from build123d import *
from build123d.topology import SkipClean

# Parameters (mm, degrees)
BOSS_EXTRUDE1_DEPTH     = 10
CUT_EXTRUDE1_DEPTH      = 29.188093475
CUT_EXTRUDE1_DEPTH_BACK = 29.188093475
SKETCH4_R               = 2.05
CUT_EXTRUDE2_OUTLINE_W  = 1.4
CUT_EXTRUDE2_OUTLINE_H  = 5.870544518
CUT_EXTRUDE3_START      = 20
CUT_EXTRUDE3_DEPTH      = 12
BOSS_EXTRUDE2_START     = 3
SKETCH8_R               = 14.5
SKETCH8_R_2             = 12.5
BOSS_EXTRUDE2_DEPTH     = 3
CUT_EXTRUDE7_DEPTH      = 3


# Read off the part's stored shape, not the designer's step: Cut-Extrude2
with BuildPart() as part:
    # Sketch1 → Boss-Extrude1 (new body)
    with BuildSketch(Plane.XY):
        with BuildLine():
            Line((-15.560899439, 8.006772674), (-9.384542241, 19.705801525))
            Line((-9.384542241, 19.705801525), (-4.384542241, 19.705801525))
            Line((-4.384542241, 19.705801525), (-4.384542241, 16.705801525))
            Line((-4.384542241, 16.705801525), (-4.384542241, 11.705801525))
            ThreePointArc((-4.384542241, 11.705801525), (0, -12.5), (4.384542241, 11.705801525))
            Line((4.384542241, 11.705801525), (4.384542241, 16.705801525))
            Line((4.384542241, 16.705801525), (4.384542241, 19.705801525))
            Line((4.384542241, 19.705801525), (9.384542241, 19.705801525))
            Line((9.384542241, 19.705801525), (15.560899439, 8.006772674))
            ThreePointArc((15.560899439, 8.006772674), (0, -17.5), (-15.560899439, 8.006772674))
        make_face()
    extrude(amount=BOSS_EXTRUDE1_DEPTH)

    # Sketch4 → Cut-Extrude1 (cut, two sides: drawn at the far end of the back side and taken through both)
    with BuildSketch(Plane(origin=(0, 0, 0), x_dir=(0, 0, -1), z_dir=(1, 0, 0)).offset(-CUT_EXTRUDE1_DEPTH_BACK)):
        with Locations(Location((-5, 14.705801525, 0), (0, 0, 90))):
            Circle(SKETCH4_R)
    extrude(amount=CUT_EXTRUDE1_DEPTH + CUT_EXTRUDE1_DEPTH_BACK, mode=Mode.SUBTRACT)

    # Cut-Extrude2 outline → Cut-Extrude2 (revolve, cut)
    with BuildSketch(Plane(origin=(0, 14.705801525, 5), x_dir=(0, 1, 0), z_dir=(0, 0, -1))):
        with Locations((2.75, -10.935272259)):
            Rectangle(CUT_EXTRUDE2_OUTLINE_W, CUT_EXTRUDE2_OUTLINE_H)
    revolve(axis=Axis((0, 14.705801525, 5), (1, 0, 0)), mode=Mode.SUBTRACT)

    # Sketch6 → Cut-Extrude3 (cut)
    with BuildSketch(Plane(origin=(0, 0, 0), x_dir=(0, 0, -1), z_dir=(1, 0, 0)).offset(CUT_EXTRUDE3_START)):
        Polygon((-1.996012472, 12.00221275), (-1.156629675, 15.955536649), (-4.160617203, 18.659125424), (-8.003987528, 17.4093903), (-8.843370325, 13.456066401), (-5.839382797, 10.752477625), align=None)
    extrude(amount=-CUT_EXTRUDE3_DEPTH, mode=Mode.SUBTRACT)

    # Sketch8 → Boss-Extrude2 (add)
    with SkipClean():  # the faces are left unmerged after this step: merging them gives an invalid solid
        with BuildSketch(Plane(origin=(0, 0, 0), x_dir=(-1, 0, 0), z_dir=(0, 0, -1)).offset(BOSS_EXTRUDE2_START)):
            with Locations(Location((0, 0, 0), (0, 0, 107.600741317))):
                Circle(SKETCH8_R)
            Circle(SKETCH8_R_2, mode=Mode.SUBTRACT)
        extrude(amount=-BOSS_EXTRUDE2_DEPTH)

    # Sketch9 → Cut-Extrude7 (cut)
    with BuildSketch(Plane.XY):
        Polygon((-4.384542241, 11.705801525), (-4.384542241, 13.821207955), (0.563137908, 18.768888104), (4.384542241, 13.821207955), (4.384542241, 11.705801525), align=None)
    extrude(amount=-CUT_EXTRUDE7_DEPTH, mode=Mode.SUBTRACT)


solid = part.part
The listing builds one solid part. Answer for the finished solid, in the listing's coordinates (mm). A direction names the side the tool comes from. Give positions to 0.01 mm unless a question says otherwise; leave off trailing zeros. Loops run counter-clockwise (first coordinate to the right, second up) from the corner with the lowest first, then second, coordinate; pieces in that order, holes last. Notation, with made-up numbers: (83, 83.5) - (142, 83.5) arc R9 cw to (142, 99.5) - close; hole circle Ø5 at (63, 41). An arc over 180 degrees is marked (long way). Answer as a JSON object with one key per item and string values.
1. Flat-ended cylindrical pins translate along their axes: pin 1 Ø1.5 at (x, z) = (-9.5, 6) entering from -Y; pin 2 Ø3.5 at (y, z) = (14.71, 5) entering from +X; pin 3 Ø2 at (x, z) = (-8, -0.5) entering from -Y; pin 4 Ø3.5 at (y, z) = (15, 5.5) entering from -X. Find the tip coordinate at first contact, or state that the pin passes through.
Determined:
{"pin 1": "y = -15.16", "pin 2": "through", "pin 3": "y = -15.98", "pin 4": "x = -8"}
2. A cutting plane is placed at A-A (z = 5). Write down the section's boundary in (x, y).
Determined:
{"outline": "(-15.56, 8.01) arc R17.5 ccw (long way) to (15.56, 8.01) - (13.97, 11.03) - (8, 11.03) - (8, 12.66) - (4.38, 12.66) - (4.38, 11.71) arc R12.5 cw (long way) to (-4.38, 11.71) - (-4.38, 12.66) - (-8, 12.66) - (-8, 11.26) - (-13.85, 11.26) - close; (-10.2, 18.16) - (-8, 18.16) - (-8, 16.76) - (-4.38, 16.76) - (-4.38, 19.71) - (-9.38, 19.71) - close; (4.38, 16.76) - (8, 16.76) - (8, 18.39) - (10.08, 18.39) - (9.38, 19.71) - (4.38, 19.71) - close"}
3. Find the intervals of material crossed by L1, parallel to Y at x = 6.9, z = 5; L2, parallel to X at y = 0, z = 5.25; L3, parallel to X at y = 0, z = -0.8, in increasing order. Write a range as [from, to].
Determined:
{"L1": "[-16.08, -10.42], [10.42, 12.66], [16.76, 19.71]", "L2": "[-17.5, -12.5], [12.5, 17.5]", "L3": "[-14.5, -12.5], [12.5, 14.5]"}
4. For faces 1 (the cylindrical face through (-10.3, 11.26, 5.15)), 2 (the flat face through (-4.385, 17, 4)), 3 (the flat face through (10.42, 12.12, 7.36)), determine the directions among +Z, -Z, +X, -X, +Y, -Y from which every point of the face is accessible in a straight line to the end or side of a thin tool.
Determined:
{"face 1": "-X", "face 2": "+Z, -Z, +Y", "face 3": "+X"}
5. A cutting plane is placed at D-D (x = 0). Write down the section's boundary in (y, z), then the cut area to 3 significant figures.
Determined:
{"outline": "(-17.5, 0) - (-14.5, 0) - (-14.5, -3) - (-12.5, -3) - (-12.5, 10) - (-17.5, 10) - close", "area": "56.0 mm²"}
6. A cutting plane is placed at C-C (y = 0). Write down the section's boundary in (x, z).
Determined:
{"outline": "(-17.5, 0) - (-14.5, 0) - (-14.5, -3) - (-12.5, -3) - (-12.5, 10) - (-17.5, 10) - close; (12.5, -3) - (14.5, -3) - (14.5, 0) - (17.5, 0) - (17.5, 10) - (12.5, 10) - close"}
7. For a pull along Z with two mould halves and no side action, classify faces 4 (the flat face through (9.854, 15.46, 8.418)), 5 (the flat face through (5, 14, 0)), 6 (the flat face through (-7, 19.706, 5)) as pulls with the +Z half, pulls with the -Z half, needs draft (parallel to the pull), parting line crosses it, or undercut.
Determined:
{"face 4": "undercut", "face 5": "pulls with the -Z half", "face 6": "needs draft"}
8. A cutting plane is placed at B-B (x = 8.5). Write down the section's boundary in (y, z), then the cut area to 3 significant figures.
Determined:
{"outline": "(-15.3, 0) - (-11.75, 0) - (-11.75, -3) - (-9.17, -3) - (-9.17, 10) - (-15.3, 10) - close; (9.17, -3) - (11.75, -3) - (11.75, 0) - (19.71, 0) - (19.71, 10) - (9.17, 10) - close; hole (10.75, 5.84) - (12, 2) - (15.96, 1.16) - (18.66, 4.16) - (17.41, 8) - (13.46, 8.84) - close", "area": "140 mm²"}
